The figure shows three views and two pictorial views of one solid part (mm, origin at its lowest corner). Answer the questions. Round coordinates to 2 decimals unless told otherwise and drop trailing zeros. Order: outer loops, then holes, each group sorted by start corner. A loop starts at its lowest first (then second) coordinate and runs counter-clockwise, first axis right, second up. Notation, with made-up numbers: (18.25, 69) -> (63.25, 69) arc R6 cw to (63.25, 75) -> close; hole circle Ø7 at (-2.75, 25). An arc over 180 degrees is marked (long way). Return JSON: item names as keys, results as strings. Group by question number.
(1) The part is cut by section A-A (z = 0.7). Determine the outline of the cut face in (x, y), plus the area to 3 significant figures.
(2) The part is cut by section C-C (x = 26). Determine the outline of the cut face in (y, z).
(3) The part is cut by section D-D (y = 15.5). Determine the outline of the cut face in (x, z) (1 decimal).
(4) This flat-tipped pin is pushed along its axis until it touches: pin 1 (4 mm diameter, centred on x = 38.99, y = 15.5, fed in from -Z). Where does it stop, or does it pass through?
(5) Consider line 1 (Y direction, x = 26, z = 1.4); line 2 (X direction, y = 14.5, z = 2.7) (1 decimal); line 3 (Y direction, x = 22, z = 0.95) (1 decimal). Determine where each line is inside the solid, lowest interval first. Write a range as [from, to].
(6) The part is cut by section B-B (y = 38). Determine the outline of the cut face in (x, z).
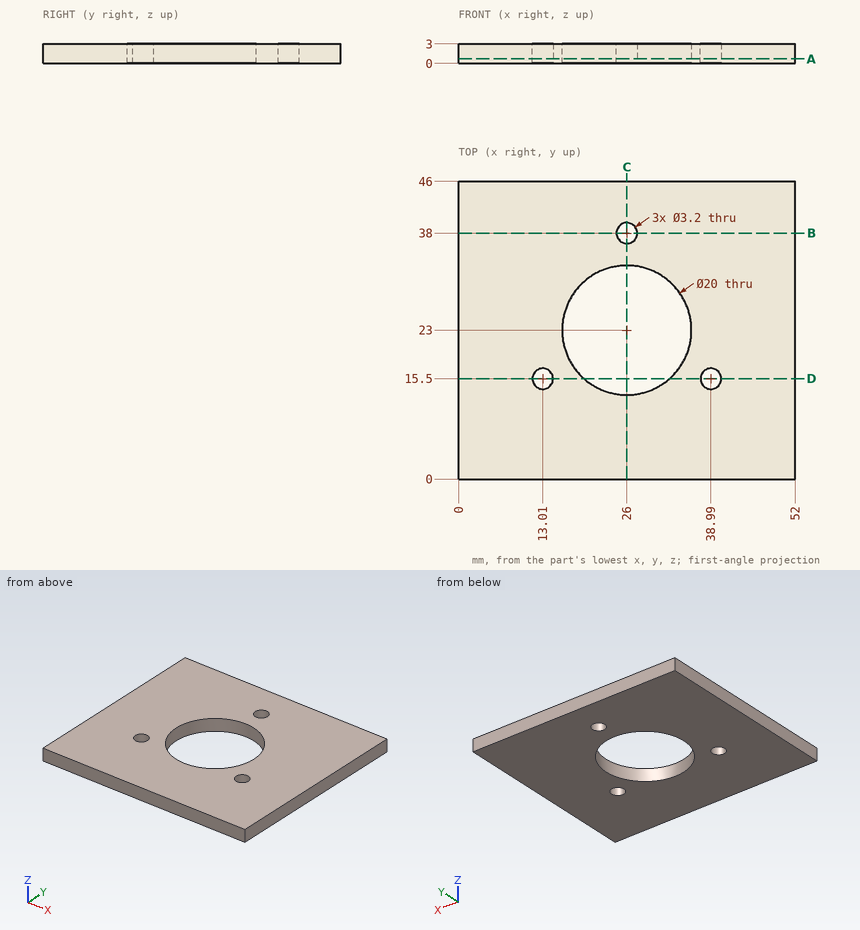
Answer below:
{
 "1": {"outline": "(0, 0) -> (52, 0) -> (52, 46) -> (0, 46) -> close; hole circle Ø3.2 at (13.01, 15.5); hole circle Ø20 at (26, 23); hole circle Ø3.2 at (26, 38); hole circle Ø3.2 at (38.99, 15.5)", "area": "2,050 mm²"},
 "2": {"outline": "(0, 0) -> (13, 0) -> (13, 3) -> (0, 3) -> close; (33, 0) -> (36.4, 0) -> (36.4, 3) -> (33, 3) -> close; (39.6, 0) -> (46, 0) -> (46, 3) -> (39.6, 3) -> close"},
 "3": {"outline": "(0, 0) -> (11.4, 0) -> (11.4, 3) -> (0, 3) -> close; (14.6, 0) -> (19.4, 0) -> (19.4, 3) -> (14.6, 3) -> close; (32.6, 0) -> (37.4, 0) -> (37.4, 3) -> (32.6, 3) -> close; (40.6, 0) -> (52, 0) -> (52, 3) -> (40.6, 3) -> close"},
 "4": {"pin 1": "stops at z = 0"},
 "5": {"line 1": "y = [0, 13], [33, 36.4], [39.6, 46]", "line 2": "x = [0, 11.8], [14.3, 20.7], [31.3, 37.7], [40.2, 52]", "line 3": "y = [0, 13.8], [32.2, 46]"},
 "6": {"outline": "(0, 0) -> (24.4, 0) -> (24.4, 3) -> (0, 3) -> close; (27.6, 0) -> (52, 0) -> (52, 3) -> (27.6, 3) -> close"}
}
